Input: part model. Units: mm. Frame: model coordinates. Face numbers are marked on the shaded views. A direction names the side the tool comes from. Round coordinates to 2 decimals unless told otherwise and drop trailing zeros. Order: outer loops, then holes, each group sorted by start corner. A loop starts at its lowest first (then second) coordinate and runs counter-clockwise, first axis right, second up. Notation, with made-up numbers: (39.25, 6) - (90.25, 6) arc R17 cw to (90.25, 18) - close; hole circle Ø6 at (-38.75, 3). An arc over 180 degrees is marked (long way). One line per item, written item: value. Start each with the question number.
from build123d import *

# Parameters (mm, degrees)
F0_W     = 216
F0_H     = 25.4
F1_DEPTH = 248
F2_R     = 7
F3_DEPTH = 12.7
F4_W     = 38
F4_H     = 50.8
F4_R     = 7
F5_DEPTH = 25.4


with BuildPart() as f1:
    # F0 (on Front) → F1 (new body)
    with BuildSketch(Plane.XZ):
        with Locations((-108, 12.7)):
            Rectangle(F0_W, F0_H)
    extrude(amount=-F1_DEPTH)

    # F2 (on face) → F3 (cut)
    with BuildSketch(Plane.XY.offset(25.4)):
        with Locations((-161, 226.081771)):
            Circle(F2_R)
        with Locations((-161, 22)):
            Circle(F2_R)
        with Locations((-23, 206)):
            Circle(F2_R)
        with Locations((-26, 53.945143)):
            Circle(F2_R)
    extrude(amount=-F3_DEPTH, mode=Mode.SUBTRACT)

    # F4 (on face) → F5 (cut, through all)
    with BuildSketch(Plane.XY.offset(25.4)):
        with Locations((-197, 124)):
            Rectangle(F4_W, F4_H)
        with Locations((-26, 53.945143)):
            Circle(F4_R)
    extrude(amount=-F5_DEPTH, mode=Mode.SUBTRACT)


solid = f1.part
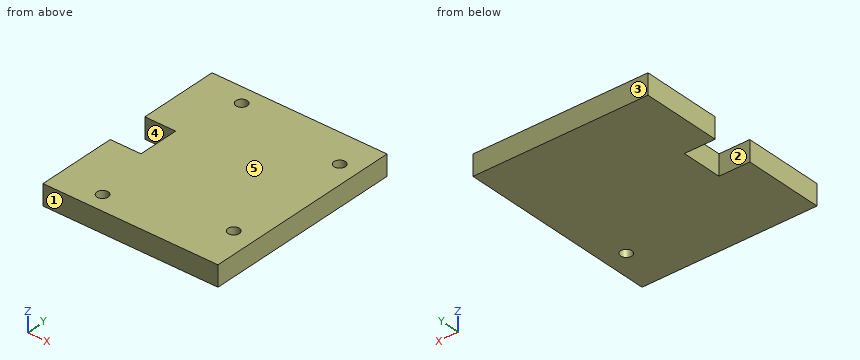
1. Section B-B (y = 206). Return the cut outline in (x, z), then the cut area to 3 significant figures.
2. Pin query (flat end, axial travel): pin 1 (5 mm diameter, centred on x = -65.5, z = 21.5, fed in from -Y); pin 2 (7 mm diameter, centred on x = -160.5, y = 223, fed in from +Z); pin 3 (12.5 mm diameter, centred on y = 122, z = 9, fed in from -X). Return the tip coordinate at first contact, or that it passes through.
3. Set-up query: the marked faces 4 and 5. Return all of +Z, -Z, +X, -X, +Y, -Y with unobstructed straight access to the full face (end or side cutting, diameter ignored); none if empty.
4. Line query: line 1 (Y direction, x = -161, z = 22.75); line 2 (Y direction, x = -183, z = 24.25); line 3 (Y direction, x = -26, z = 19.5). Output: solid intervals per line, ascending. Write a range as from..to.
5. Pull-direction query (Y, two-part tool) for the marked faces 1, 2 and 3; classes: released by +Y, released by -Y, zero draft, split by the parting line, or undercut.
6. Section A-A (x = -23). Return the cut outline in (y, z), then the cut area to 3 significant figures.
7. Section C-C (z = 5.5). Return the cut outline in (x, y), then the cut area to 3 significant figures.
8. Section D-D (x = -161). Return the cut outline in (y, z).
Solved:
1. outline: (-216, 0) - (0, 0) - (0, 25.4) - (-16, 25.4) - (-16, 12.7) - (-30, 12.7) - (-30, 25.4) - (-216, 25.4) - close
1. area: 5,310 mm²
2. pin 1: stops at y = 0
2. pin 2: stops at z = 12.7
2. pin 3: stops at x = -178
3. face 4: +Z, -Z, -X
3. face 5: +Z, +X, -X, +Y, -Y
4. line 1: y = 0..15, 29..219.08, 233.08..248
4. line 2: y = 0..98.6, 149.4..248
4. line 3: y = 0..46.95, 60.95..199.68, 212.32..248
5. face 1: released by -Y
5. face 2: undercut
5. face 3: released by +Y
6. outline: (0, 0) - (47.62, 0) - (47.62, 25.4) - (0, 25.4) - close; (60.27, 0) - (248, 0) - (248, 25.4) - (213, 25.4) - (213, 12.7) - (199, 12.7) - (199, 25.4) - (60.27, 25.4) - close
6. area: 5,800 mm²
7. outline: (-216, 0) - (0, 0) - (0, 248) - (-216, 248) - (-216, 149.4) - (-178, 149.4) - (-178, 98.6) - (-216, 98.6) - close; hole circle Ø14 at (-26, 53.95)
7. area: 51,500 mm²
8. outline: (0, 0) - (248, 0) - (248, 25.4) - (233.08, 25.4) - (233.08, 12.7) - (219.08, 12.7) - (219.08, 25.4) - (29, 25.4) - (29, 12.7) - (15, 12.7) - (15, 25.4) - (0, 25.4) - close
